The model under review builds one solid part; all positions refer to its coordinate system, in mm. Coordinates: 2 decimals unless noted, no trailing zeros. Write each loop counter-clockwise with the first axis right and the second up, starting at its lowest first coordinate (ties: lowest second). Pieces come first, ordered by that corner, then holes. Notation, with made-up numbers: (-21, 39) - (22, 39) arc R8 cw to (22, 49) - close; hole circle Ø4 at (27, 9). An arc over 180 degrees is marked (long way). Return JSON: item names as keys, results as strings. Group by question number.
(1) Draft analysis for pull direction X (two halves, no side actions). For faces 1 (the face through (3.013, 2.267, 2.252)), 2 (the face through (-6, 0, 2)), state which applies: released by +X, released by -X, zero draft, split by the parting line, or undercut.
(2) We need section A-A on x = 5.25. State the section outline as (y, z) points.
(3) For pin 1 Ø1.5 at (x, z) = (-1, 3) entering from +Y; pin 2 Ø1.5 at (y, z) = (-1, 0.5) entering from +X; pin 3 Ø1.5 at (x, z) = (-4, 3) entering from -Y, all flat-tipped, find the tip position at first contact; note any pin that passes through.
(4) To check wall thickness, follow L1, parallel to X at y = 1, z = 2.2; L2, parallel to Y at x = -1.75, z = 4.3; L3, parallel to X at y = -4, z = 3.6. State the ranges of each line that lie inside material, in increasing order. Write a range as from..to.
```python
from build123d import *

# Parameters (mm, degrees)
SKETCH1_R                          = 6
SKETCH1_R_2                        = 4.075
RING_DEPTH                         = 5
SINGLE_TEETH_DEPTH                 = 5
TEETHCHAMPFER_SIZE                 = 0.25
TEETHCHAMPFER_SIZE2                = 0.433012702
F_15TH_TEETHS_COUNT                = 15
TEETHCHAMPFER_OF_15TH_TEETHS_SIZE2 = 0.433012702
TEETHCHAMPFER_OF_15TH_TEETHS_SIZE  = 0.25


with BuildPart() as part:
    # Sketch1 → ring (new body)
    with BuildSketch(Plane.XY):
        Circle(SKETCH1_R)
        Circle(SKETCH1_R_2, mode=Mode.SUBTRACT)
    extrude(amount=RING_DEPTH)

    # Sketch1<4> → single teeth (add)
    with BuildSketch(Plane.XY):
        with BuildLine():
            Line((-0.673142232, 4.019017857), (0, 3.5))
            Line((0, 3.5), (0.673142232, 4.019017857))
            ThreePointArc((0.673142232, 4.019017857), (0, 4.075), (-0.673142232, 4.019017857))
        make_face()
    single_teeth = extrude(amount=SINGLE_TEETH_DEPTH)

    # teethChampfer
    teethchampfer_edges = [part.edges().sort_by_distance(p)[0] for p in [
        (-0.336571116, 3.759508929, 5),
        (0.336571116, 3.759508929, 5),
    ]]
    teethchampfer_side = [part.faces().sort_by_distance(p)[0] for p in [
        (-5.830294373, 0, 5),
    ]]
    chamfer(teethchampfer_edges, length=TEETHCHAMPFER_SIZE, length2=TEETHCHAMPFER_SIZE2, reference=teethchampfer_side[0])

    # 15th teeths: single teeth ×15 about axis
    f_15th_teeths_axis = Axis((0, 0, 0), (0, 0, 1))
    for i in range(1, F_15TH_TEETHS_COUNT):
        add(single_teeth.rotate(f_15th_teeths_axis, i * 360 / F_15TH_TEETHS_COUNT))

    # teethChampfer of 15th teeths
    teethchampfer_of_15th_teeths_edges = [part.edges().sort_by_distance(p)[0] for p in [
        (-1.836603055, 3.297586499, 5),
        (-1.221657027, 3.57137811, 5),
        (-3.019069641, 2.265481406, 5),
        (-2.568649572, 2.765723572, 5),
        (-3.679511659, 0.841653997, 5),
        (-3.47149927, 1.481850302, 5),
        (-3.703732684, -0.727703035, 5),
        (-3.774095207, -0.058248347, 5),
        (-3.08754468, -2.171233601, 5),
        (-3.424115796, -1.588275328, 5),
        (-1.937492152, -3.239338152, 5),
        (-2.482075657, -2.843675076, 5),
        (-0.452429629, -3.747331708, 5),
        (-1.110862087, -3.607377569, 5),
        (1.110862087, -3.607377569, 5),
        (0.452429629, -3.747331708, 5),
        (2.482075657, -2.843675076, 5),
        (1.937492152, -3.239338152, 5),
        (3.424115796, -1.588275328, 5),
        (3.08754468, -2.171233601, 5),
        (3.774095207, -0.058248347, 5),
        (3.703732684, -0.727703035, 5),
        (3.47149927, 1.481850302, 5),
        (3.679511659, 0.841653997, 5),
        (2.568649572, 2.765723572, 5),
        (3.019069641, 2.265481406, 5),
        (1.221657027, 3.57137811, 5),
        (1.836603055, 3.297586499, 5),
    ]]
    chamfer(teethchampfer_of_15th_teeths_edges, length=TEETHCHAMPFER_OF_15TH_TEETHS_SIZE, length2=TEETHCHAMPFER_OF_15TH_TEETHS_SIZE2)


solid = part.part
```
Ans:
{
 "1": {"face 1": "undercut", "face 2": "split by the parting line"},
 "2": {"outline": "(-2.9, 0) - (2.9, 0) - (2.9, 5) - (-2.9, 5) - close"},
 "3": {"pin 1": "y = 5.99", "pin 2": "x = 5.99", "pin 3": "y = -5.04"},
 "4": {"L1": "-5.92..-3.45, 3.45..5.92", "L2": "-5.74..-3.68, 3.28..5.74", "L3": "-4.47..-0.24, 0.24..4.47"}
}
